```python
from build123d import *

# Parameters (mm, degrees)
SKETCH3_W           = 40
SKETCH3_H           = 27
SKETCH3_R           = 2.55
BOSS_EXTRUDE1_DEPTH = 3
CUT_EXTRUDE1_DEPTH  = 1
SKETCH5_W           = 3
SKETCH5_H           = 26
CUT_EXTRUDE2_DEPTH  = 1.2
SKETCH6_R           = 1.025
CUT_EXTRUDE3_DEPTH  = 3


with BuildPart() as part:
    # Sketch3 → Boss-Extrude1 (new body)
    with BuildSketch(Plane.XY):
        Rectangle(SKETCH3_W, SKETCH3_H)
        with Locations((-15, 0)):
            Circle(SKETCH3_R, mode=Mode.SUBTRACT)
        with Locations((15, 0)):
            Circle(SKETCH3_R, mode=Mode.SUBTRACT)
    extrude(amount=BOSS_EXTRUDE1_DEPTH)

    # Sketch4 → Cut-Extrude1 (cut)
    with BuildSketch(Plane.XY.offset(3)):
        Polygon((-8, 13), (-8, -13), (8, -13), (8, 13), (2.5, 13), (2.5, 13.5), (-2.5, 13.5), (-2.5, 13), align=None)
    extrude(amount=-CUT_EXTRUDE1_DEPTH, mode=Mode.SUBTRACT)

    # Sketch5 → Cut-Extrude2 (cut)
    with BuildSketch(Plane.XY.offset(2)):
        with Locations((6.5, 0)):
            Rectangle(SKETCH5_W, SKETCH5_H)
    extrude(amount=-CUT_EXTRUDE2_DEPTH, mode=Mode.SUBTRACT)

    # Sketch6 → Cut-Extrude3 (cut)
    with BuildSketch(Plane.XY.offset(2)):
        with Locations((-5.5, 10.25)):
            Circle(SKETCH6_R)
        with Locations((-5.5, -10.25)):
            Circle(SKETCH6_R)
    extrude(amount=-CUT_EXTRUDE3_DEPTH, mode=Mode.SUBTRACT)


solid = part.part
```
Model file for the job. Use its own axes, mm. A direction names the side the tool comes from. Coordinates: 2 decimals unless noted, no trailing zeros. Write each loop counter-clockwise with the first axis right and the second up, starting at its lowest first coordinate (ties: lowest second). Pieces come first, ordered by that corner, then holes. Notation, with made-up numbers: (36, -34) - (75, -34) arc R28 ccw to (75, -9) - close; hole circle Ø7 at (8, -24). An arc over 180 degrees is marked (long way). Use a Markdown table: item, result. Add a question column.
Item 1: Drop flat-ended pins along their axis: pin 1 (6.5 mm diameter, centred on x = -0.5, y = 4.5, fed in from +Z); pin 2 (1.5 mm diameter, centred on x = 6, y = 1.5, fed in from +Z). Give the stop position or say it passes through.
Item 2: Band-saw the part on B-B, the plane x = -15. Write the cut outline in (y, z), and give its area (3 significant figures).
Item 3: Two-plate mould, pull along X, no slides. Class faces 3 (the face through (-8, 0.2, 2.5)), 4 (the face through (-9, 0, 3)), 5 (the face through (20, 0, 1)), 6 (the face through (-20, 0, 1)): pulls with the +X half, pulls with the -X half, needs draft (parallel to the pull), parting line crosses it, or undercut.
Item 4: Band-saw the part on D-D, the plane y = -10.25. Write the cut outline in (x, z) (3 decimals), and give its area (3 significant figures).
Item 5: 3-axis set-ups, long thin cutter, end or side, ignore diameter. For faces 1 (the face through (-5.2, 13, 2.5)), 2 (the face through (-6.524, -10.205, 1.014)): which of +Z, -Z, +X, -X, +Y, -Y reach the whole face in a straight line?
Item 6: Band-saw the part on A-A, the plane y = 0. Write the cut outline in (x, z).
Item 7: Drill centre lines: line 1 along X through (y, z) = (7, 2.5); line 2 along X through (y, z) = (8, 1.25); line 3 along Y through (x, z) = (15, 2.3). Where is each one in solid material? Low to high.
Item 8: Band-saw the part on C-C, the plane z = 0.4. Write the cut outline in (x, y) (3 decimals), and give its area (3 significant figures).
A:
| question | item | result |
|---|---|---|
| 1 | pin 1 | stops at z = 2 |
| 1 | pin 2 | stops at z = 0.8 |
| 2 | outline | (-13.5, 0) - (-2.55, 0) - (-2.55, 3) - (-13.5, 3) - close; (2.55, 0) - (13.5, 0) - (13.5, 3) - (2.55, 3) - close |
| 2 | area | 65.7 mm² |
| 3 | face 3 | undercut |
| 3 | face 4 | needs draft |
| 3 | face 5 | pulls with the +X half |
| 3 | face 6 | pulls with the -X half |
| 4 | outline | (-20, 0) - (-6.525, 0) - (-6.525, 2) - (-8, 2) - (-8, 3) - (-20, 3) - close; (-4.475, 0) - (20, 0) - (20, 3) - (8, 3) - (8, 0.8) - (5, 0.8) - (5, 2) - (-4.475, 2) - close |
| 4 | area | 96.3 mm² |
| 5 | face 1 | +Z |
| 5 | face 2 | +Z, -Z |
| 6 | outline | (-20, 0) - (-17.55, 0) - (-17.55, 3) - (-20, 3) - close; (-12.45, 0) - (12.45, 0) - (12.45, 3) - (8, 3) - (8, 0.8) - (5, 0.8) - (5, 2) - (-8, 2) - (-8, 3) - (-12.45, 3) - close; (17.55, 0) - (20, 0) - (20, 3) - (17.55, 3) - close |
| 7 | line 1 | x = -20 to -8, 8 to 20 |
| 7 | line 2 | x = -20 to 5, 8 to 20 |
| 7 | line 3 | y = -13.5 to -2.55, 2.55 to 13.5 |
| 8 | outline | (-20, -13.5) - (20, -13.5) - (20, 13.5) - (-20, 13.5) - close; hole circle Ø5.1 at (-15, 0); hole circle Ø2.05 at (-5.5, -10.25); hole circle Ø2.05 at (-5.5, 10.25); hole circle Ø5.1 at (15, 0) |
| 8 | area | 1,030 mm² |
